CAD build for the part. Positions are in the model's coordinates, mm. Face numbers are marked on the shaded views. A direction names the side the tool comes from. Coordinates: 2 decimals unless noted, no trailing zeros. Loops run counter-clockwise (first coordinate to the right, second up) from the corner with the lowest first, then second, coordinate; pieces in that order, holes last. Notation, with made-up numbers: (-11.75, 57) -> (39.25, 57) arc R20 cw to (39.25, 89) -> close; hole circle Ø6 at (3, -40). An arc over 180 degrees is marked (long way). Return JSON: item names as keys, results as strings. Group by question number.
(1) Flat gauge pins, fed straight in: pin 1 Ø1.5 at (y, z) = (12.5, -7) entering from -X; pin 2 Ø5.5 at (y, z) = (17, 7.5) entering from -X; pin 3 Ø4 at (x, y) = (-10.5, 29) entering from -Z; pin 4 Ø8 at (y, z) = (27.5, 7.5) entering from -X. Where does each tip first touch, or does it go through?
(2) Saw through at C-C on z = 9. Give the number of separate pieces and of enclosed holes in the cut face, then the cut area to 3 significant figures.
(3) Probe L1, parallel to X at y = 14, z = 0; L2, parallel to Y at x = -0.5, z = -23.5; L3, parallel to X at y = 2, z = 10. List the from-to ranges inside material, lowest first.
(4) Saw through at A-A on x = 0. Write the cut outline in (y, z).
(5) Mould opens along Z. For the marked faces 6, 7 and 8 say: pulls with the +Z half, pulls with the -Z half, needs draft (parallel to the pull), parting line crosses it, or undercut.
(6) Saw through at B-B on z = -1. Write the cut outline in (x, y).
(7) Tool access for the marked faces 1, 2, 3, 4 and 5: list every direction of +Z, -Z, +X, -X, +Y, -Y with a clear straight run to the whole face (end or side of a thin tool).
(8) Saw through at D-D on x = -18. Write the cut outline in (y, z), then the cut area to 3 significant figures.
```python
from build123d import *

# Parameters (mm, degrees)
ESQUISSE5_R             = 2.5
BOSS_EXTRU_2_DEPTH      = 5
ESQUISSE6_R             = 7.5
BOSS_EXTRU_3_DEPTH      = 30
BOSS_EXTRU_6_START      = -15
BOSS_EXTRU_6_DEPTH      = 15
ESQUISSE14_R            = 3.95
ENL_V_MAT_EXTRU_4_DEPTH = 52.800900893
ENL_V_MAT_EXTRU_5_DEPTH = 25
CONG_2_R                = 3
ESQUISSE17_R            = 2.5
ENL_V_MAT_EXTRU_6_DEPTH = 53.189940485
ENL_V_MAT_EXTRU_7_DEPTH = 4.5


with BuildPart() as part:
    # Esquisse5 → Boss.-Extru.2 (new body)
    with BuildSketch(Plane(origin=(0, 0, 0), x_dir=(1, 0, 0), z_dir=(0, 1, 0))):
        Polygon((-25, -14.43375673), (25, -14.43375673), (0, 28.867513459), align=None)
        with Locations(Location((0, 20, 0), (0, 0, 270))):
            Circle(ESQUISSE5_R, mode=Mode.SUBTRACT)
        with Locations(Location((-17.320508076, -10, 0), (0, 0, 270))):
            Circle(ESQUISSE5_R, mode=Mode.SUBTRACT)
        with Locations(Location((17.320508076, -10, 0), (0, 0, 270))):
            Circle(ESQUISSE5_R, mode=Mode.SUBTRACT)
    extrude(amount=BOSS_EXTRU_2_DEPTH)

    # Esquisse6 → Boss.-Extru.3 (add)
    with BuildSketch(Plane(origin=(0, 5, 0), x_dir=(1, 0, 0), z_dir=(0, 1, 0))):
        with Locations(Location((0, 0, 0), (0, 0, 270))):
            Circle(ESQUISSE6_R)
    extrude(amount=BOSS_EXTRU_3_DEPTH)

    # Esquisse13 → Boss.-Extru.6 (add)
    with BuildSketch(Plane(origin=(0, 35, 0), x_dir=(1, 0, 0), z_dir=(0, 1, 0)).offset(BOSS_EXTRU_6_START)):
        with BuildLine():
            Line((-6, -4.5), (-6, -14.5))
            Line((-6, -14.5), (6, -14.5))
            Line((6, -14.5), (6, -4.5))
            ThreePointArc((6, -4.5), (0, -7.5), (-6, -4.5))
        make_face()
    extrude(amount=BOSS_EXTRU_6_DEPTH)

    # Esquisse14 → Enlèv. mat.-Extru.4 (cut, through all)
    with BuildSketch(Plane(origin=(0, 35, 0), x_dir=(1, 0, 0), z_dir=(0, 1, 0))):
        with Locations(Location((0, 0, 0), (0, 0, 270))):
            Circle(ESQUISSE14_R)
    extrude(amount=-ENL_V_MAT_EXTRU_4_DEPTH, mode=Mode.SUBTRACT)

    # Esquisse15 → Enlèv. mat.-Extru.5 (cut)
    with BuildSketch(Plane(origin=(0, 35, 0), x_dir=(1, 0, 0), z_dir=(0, 1, 0))):
        with BuildLine():
            Line((-1, -3.821321761), (-1, -14.5))
            Line((-1, -14.5), (1, -14.5))
            Line((1, -14.5), (1, -3.821321761))
            ThreePointArc((1, -3.821321761), (0, -3.95), (-1, -3.821321761))
        make_face()
    extrude(amount=-ENL_V_MAT_EXTRU_5_DEPTH, mode=Mode.SUBTRACT)

    # Congé2
    cong_2_edges = [part.edges().sort_by_distance(p)[0] for p in [
        (0, 2.5, -28.867513459),
        (25, 2.5, 14.43375673),
        (-25, 2.5, 14.43375673),
    ]]
    fillet(cong_2_edges, radius=CONG_2_R)

    # Esquisse17 → Enlèv. mat.-Extru.6 (cut, through all)
    with BuildSketch(Plane(origin=(6, 0, 0), x_dir=(0, 0, -1), z_dir=(1, 0, 0))):
        with Locations(Location((-9.5, 27.5, 0), (0, 0, 180))):
            Circle(ESQUISSE17_R)
    extrude(amount=-ENL_V_MAT_EXTRU_6_DEPTH, mode=Mode.SUBTRACT)

    # Esquisse18 → Enlèv. mat.-Extru.7 (cut)
    with BuildSketch(Plane.ZY.offset(6)):
        Polygon((11.786307066, 31.46), (7.213692934, 31.46), (4.927385868, 27.5), (7.213692934, 23.54), (11.786307066, 23.54), (14.072614132, 27.5), align=None)
    extrude(amount=-ENL_V_MAT_EXTRU_7_DEPTH, mode=Mode.SUBTRACT)


solid = part.part
```
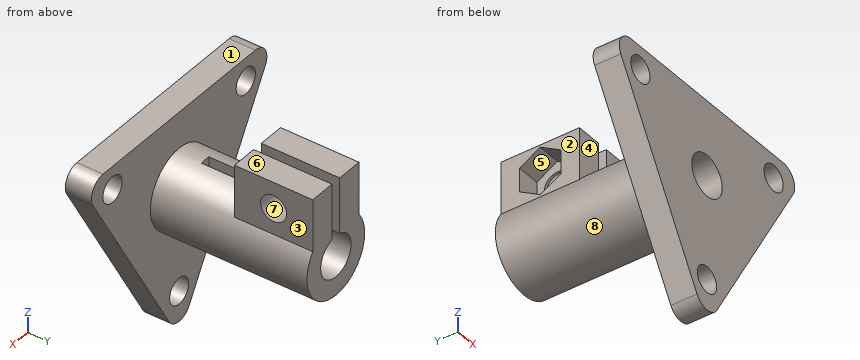
Geometry results:
{
 "1": {"pin 1": "x = -4.15", "pin 2": "x = -5.8", "pin 3": "through", "pin 4": "x = -6.63"},
 "2": {"separate pieces": "7", "enclosed holes": "0", "area": "260 mm²"},
 "3": {"L1": "-7.5 to -3.95, 3.95 to 7.5", "L2": "0 to 5", "L3": "-22.44 to -19.82, -14.82 to 14.82, 19.82 to 22.44"},
 "4": {"outline": "(0, -25.87) -> (5, -25.87) -> (5, -22.5) -> (0, -22.5) -> close; (0, -17.5) -> (5, -17.5) -> (5, -7.5) -> (35, -7.5) -> (35, -3.95) -> (0, -3.95) -> close; (0, 3.95) -> (10, 3.95) -> (10, 7.5) -> (5, 7.5) -> (5, 14.43) -> (0, 14.43) -> close"},
 "5": {"face 6": "pulls with the +Z half", "face 7": "undercut", "face 8": "parting line crosses it"},
 "6": {"outline": "(-16.09, 0) -> (-3.82, 0) -> (-3.82, 35) -> (-7.43, 35) -> (-7.43, 5) -> (-16.09, 5) -> close; (3.82, 0) -> (16.09, 0) -> (16.09, 5) -> (7.43, 5) -> (7.43, 35) -> (3.82, 35) -> close"},
 "7": {"face 1": "+Z, +X, -X, -Y", "face 2": "+Z, -X, +Y", "face 3": "+Z, +X, +Y", "face 4": "+Z, -X", "face 5": "-X"},
 "8": {"outline": "(0, 2.31) -> (5, 2.31) -> (5, 7.59) -> (0, 7.59) -> close; (0, 12.41) -> (5, 12.41) -> (5, 14.43) -> (0, 14.43) -> close", "area": "36.6 mm²"}
}
